from build123d import *

# Parameters (mm, degrees)
SKETCH004_R  = 7.5
PAD004_DEPTH = 10
FILLET_R     = 0.5
SKETCH005_R  = 2.7
PAD005_DEPTH = 1
SKETCH006_R  = 0.75
PAD006_DEPTH = 0.5
FILLET001_R  = 0.2


with BuildPart() as part:
    # Sketch004 → Pad004 (new body)
    with BuildSketch(Plane.XY):
        Circle(SKETCH004_R)
    extrude(amount=-PAD004_DEPTH)

    # Fillet
    fillet_edges = [part.edges().sort_by_distance(p)[0] for p in [
        (-7.5, 0, 0),
        (-7.5, 0, -10),
    ]]
    fillet(fillet_edges, radius=FILLET_R)

    # Sketch005 (on Face5 of Fillet) → Pad005 (join)
    with BuildSketch(Plane(origin=(0, 0, -10), x_dir=(1, 0, 0), z_dir=(0, 0, -1))):
        Circle(SKETCH005_R)
    extrude(amount=PAD005_DEPTH)

    # Sketch006 (on Face7 of Pad005) → Pad006 (join)
    with BuildSketch(Plane(origin=(0, 0, -11), x_dir=(1, 0, 0), z_dir=(0, 0, -1))):
        Circle(SKETCH006_R)
    extrude(amount=PAD006_DEPTH)

    # Fillet001
    fillet001_edges = [part.edges().sort_by_distance(p)[0] for p in [
        (-0.75, 0, -11.5),
    ]]
    fillet(fillet001_edges, radius=FILLET001_R)


solid = part.part
For this review, take the finished solid that the model builds, in its own axes (mm). A direction names the side the tool comes from. Round coordinates to 2 decimals unless told otherwise and drop trailing zeros. Loops run counter-clockwise (first coordinate to the right, second up) from the corner with the lowest first, then second, coordinate; pieces in that order, holes last. Notation, with made-up numbers: (-25.5, 63.25) - (-14.5, 63.25) arc R8 cw to (-14.5, 74.25) - close; hole circle Ø6 at (-13.75, 68). An arc over 180 degrees is marked (long way). Use one line per item in the form item = value.
Item 1: For line 1 (Y direction, x = -0.25, z = -9); line 2 (Z direction, x = -0.25, y = -4.25); line 3 (Z direction, x = 2.25, y = 0.5), list the stretches that pass through material, from the lowest coordinate up.
Answers:
line_1 = -7.5 to 7.5
line_2 = -10 to 0
line_3 = -11 to 0
Item 2: Clearance check with flat-ended pins moving along their axes: P1, Ø8, axis at x = -3.5, y = -0.5, coming from the +Z side; P2, Ø5, axis at x = 0, y = -5, coming from the -Z side; P3, Ø2, axis at y = -4.5, z = -9.5, coming from the -X side; P4, Ø1.5, axis at y = -3.5, z = -3.5, coming from the +X side. State where each tip first meets the part, or that it passes through.
Answers:
P1 = 0
P2 = -11
P3 = -6.63
P4 = 6.98
Item 3: Consider section A-A on x = 0. Write out the cut boundary in (y, z), then the cut area to 3 significant figures.
Answers:
outline = (-7.5, -9.5) arc R0.5 ccw to (-7, -10) - (-2.7, -10) - (-2.7, -11) - (-0.75, -11) - (-0.75, -11.3) arc R0.2 ccw to (-0.55, -11.5) - (0.55, -11.5) arc R0.2 ccw to (0.75, -11.3) - (0.75, -11) - (2.7, -11) - (2.7, -10) - (7, -10) arc R0.5 ccw to (7.5, -9.5) - (7.5, -0.5) arc R0.5 ccw to (7, 0) - (-7, 0) arc R0.5 ccw to (-7.5, -0.5) - close
area = 156 mm^2
Item 4: Consider section C-C on z = -8.5. Write out the cut boundary in (x, y), then the cut area to 3 significant figures.
Answers:
outline = circle Ø15 at (0, 0)
area = 177 mm^2
Item 5: Tool access review of faces 1 (the cylindrical face through (-0.75, -0.03, -11.15)), 2 (the flat face through (0, 0, 0)): name each direction out of +Z, -Z, +X, -X, +Y, -Y from which nothing blocks a thin tool from reaching the whole face with its end or side.
Answers:
face_1 = -Z
face_2 = +Z, +X, -X, +Y, -Y
